Build history of the part. All positions in model axes, mm. A direction names the side the tool comes from. Give positions to 0.01 mm unless a question says otherwise; leave off trailing zeros. Loops run counter-clockwise (first coordinate to the right, second up) from the corner with the lowest first, then second, coordinate; pieces in that order, holes last. Notation, with made-up numbers: (40.5, 89.25) -> (46.5, 89.25) arc R30 cw to (46.5, 115.25) -> close; hole circle Ø7 at (39.5, -23). An arc over 180 degrees is marked (long way). Answer as a JSON object with one key per item and string values. Group by question number.
Q1. Band-saw the part on B-B, the plane z = 17. Count the separate pieces of the cut face and the enclosed holes in it, plus the area to 3 significant figures.
Q2. Two-plate mould, pull along X, no slides. Class faces 1 (the flat face through (112.867, -11, 13)), 2 (the flat face through (57.2, -26.2, 12.5)), 3 (the flat face through (127, -42, 25.4)), 4 (the cylindrical face through (-0.831, 67.892, 30.244)): pulls with the +X half, pulls with the -X half, needs draft (parallel to the pull), parting line crosses it, or undercut.
Q3. Wall check: probe 1 along Z at (x, y) = (220, -45.5); probe 2 along Y at (x, z) = (127.5, 11); probe 3 along Y at (x, z) = (140, 21). Give the ranges that are in metal, low to high. Write a range as from..to.
Q4. Drop flat-ended pins along their axis: pin 1 (20.5 mm diameter, centred on y = 0, z = 10.5, fed in from -X); pin 2 (8 mm diameter, centred on x = 116.5, z = 21, fed in from -Y); pin 3 (1.4 mm diameter, centred on y = -30.5, z = 15, fed in from +X); pin 4 (12 mm diameter, centred on x = 196, z = 32.5, fed in from -Y). Give the stop position or say it passes through.
Q5. Tool access for faces 5 (the flat face through (164, -42, 0)), 6 (the flat face through (230.488, -22, 13)), 7 (the flat face through (0, 0, 0)): list every direction of +Z, -Z, +X, -X, +Y, -Y with a clear straight run to the whole face (end or side of a thin tool).
Q6. Band-saw the part on C-C, the plane x = 234.5. Write the cut outline in (y, z), plus the area to 3 significant figures.
Q7. Band-saw the part on A-A, the plane x = 0. Write the cut outline in (y, z).
from build123d import *

# Parameters (mm, degrees)
F1_R     = 6.379673691
F3_W     = 4.8832285095
F3_H     = 45.7555688669
F3_H_2   = 32.2255445958
F4_DEPTH = 25.4
F6_DEPTH = 25.4


with BuildPart() as f2:
    # F2: sweep along a path in F0
    with BuildLine(Plane.YZ) as f2_path:
        Line((0, 0), (48.8668594837, 0))
        ThreePointArc((48.8668594837, 0), (57.8471156048, 3.7197438789), (61.5668594837, 12.7))
        Line((61.5668594837, 12.7), (61.5668594837, 47.304409945))
        ThreePointArc((61.5668594837, 47.304409945), (65.2866033626, 56.2846660661), (74.2668594837, 60.004409945))
        Line((74.2668594837, 60.004409945), (106.4591375947, 60.004409945))
    # F1 (on Front) → F2 (sweep)
    with BuildSketch(Plane.XZ):
        Circle(F1_R)
    sweep(path=f2_path.line)

    # F3 (on Top) → F4 (join)
    with BuildSketch(Plane.XY):
        Polygon((326.6327083111, 18.4751711786), (4.1886316997, 19.5212387724), (90.2807963532, -142.4016799862), align=None)
        Polygon((87.5756415589, -33.0956764519), (82.4007365874, -33.0956764519), (77.0470621713, -19.4245184088), (59.819333075, -19.4245184088), (54.5315210859, -33.0956764519), (49.4695231318, -33.0956764519), (66.4620292749, 10.0724399292), (70.6678156791, 10.0724399292), align=None, mode=Mode.SUBTRACT)
        with Locations((95.1921607853, -10.2178920185)):
            Rectangle(F3_W, F3_H, mode=Mode.SUBTRACT)
        with Locations((110.425199238, -10.2178920185)):
            Rectangle(F3_W, F3_H, mode=Mode.SUBTRACT)
        with Locations((125.6582376907, -16.982904154)):
            Rectangle(F3_W, F3_H_2, mode=Mode.SUBTRACT)
        with BuildLine():
            add(Edge.make_bspline(
                [(157.2204535583, -18.9822992567), (159.2339620381, -21.099305836), (159.2339620381, -24.3077469184)],
                knots=[0, 0, 0, 1, 1, 1], degree=2))
            add(Edge.make_bspline(
                [(159.2339620381, -24.3077469184), (159.2339620381, -28.8052097846), (155.8843871838, -31.2468240393)],
                knots=[0, 0, 0, 1, 1, 1], degree=2))
            add(Edge.make_bspline(
                [(155.8843871838, -31.2468240393), (152.5348123295, -33.6884382941), (146.4754690537, -33.6884382941)],
                knots=[0, 0, 0, 1, 1, 1], degree=2))
            add(Edge.make_bspline(
                [(146.4754690537, -33.6884382941), (140.067995807, -33.6884382941), (136.4831979994, -31.656111978)],
                knots=[0, 0, 0, 1, 1, 1], degree=2))
            Line((136.4831979994, -31.656111978), (136.4831979994, -27.1304223574))
            add(Edge.make_bspline(
                [(136.4831979994, -27.1304223574), (138.8072007776, -28.3065371237), (141.4652201494, -28.97927477)],
                knots=[0, 0, 0, 1, 1, 1], degree=2))
            add(Edge.make_bspline(
                [(141.4652201494, -28.97927477), (144.1232395211, -29.6520124163), (146.5977849894, -29.6520124163)],
                knots=[0, 0, 0, 1, 1, 1], degree=2))
            add(Edge.make_bspline(
                [(146.5977849894, -29.6520124163), (150.4178057502, -29.6520124163), (152.4736543616, -28.4335575184)],
                knots=[0, 0, 0, 1, 1, 1], degree=2))
            add(Edge.make_bspline(
                [(152.4736543616, -28.4335575184), (154.5295029731, -27.2151026206), (154.5295029731, -24.712330398)],
                knots=[0, 0, 0, 1, 1, 1], degree=2))
            add(Edge.make_bspline(
                [(154.5295029731, -24.712330398), (154.5295029731, -22.8305467719), (152.9017601366, -21.4944803975)],
                knots=[0, 0, 0, 1, 1, 1], degree=2))
            add(Edge.make_bspline(
                [(152.9017601366, -21.4944803975), (151.2740173, -20.158414023), (146.5319225624, -18.3330839057)],
                knots=[0, 0, 0, 1, 1, 1], degree=2))
            add(Edge.make_bspline(
                [(146.5319225624, -18.3330839057), (142.0344596962, -16.6582964786), (140.138562693, -15.4069103672)],
                knots=[0, 0, 0, 1, 1, 1], degree=2))
            add(Edge.make_bspline(
                [(140.138562693, -15.4069103672), (138.2426656898, -14.1555242559), (137.315887254, -12.570121551)],
                knots=[0, 0, 0, 1, 1, 1], degree=2))
            add(Edge.make_bspline(
                [(137.315887254, -12.570121551), (136.3891088181, -10.9847188461), (136.3891088181, -8.7830320036)],
                knots=[0, 0, 0, 1, 1, 1], degree=2))
            add(Edge.make_bspline(
                [(136.3891088181, -8.7830320036), (136.3891088181, -4.8406953071), (139.5975499005, -2.5590326605)],
                knots=[0, 0, 0, 1, 1, 1], degree=2))
            add(Edge.make_bspline(
                [(139.5975499005, -2.5590326605), (142.8059909829, -0.277370014), (148.3854794341, -0.277370014)],
                knots=[0, 0, 0, 1, 1, 1], degree=2))
            add(Edge.make_bspline(
                [(148.3854794341, -0.277370014), (153.5886111601, -0.277370014), (158.5659288509, -2.3943765933)],
                knots=[0, 0, 0, 1, 1, 1], degree=2))
            Line((158.5659288509, -2.3943765933), (156.8252789968, -6.3649400442))
            add(Edge.make_bspline(
                [(156.8252789968, -6.3649400442), (151.9796861598, -4.3702494006), (148.0373494633, -4.3702494006)],
                knots=[0, 0, 0, 1, 1, 1], degree=2))
            add(Edge.make_bspline(
                [(148.0373494633, -4.3702494006), (144.5654586732, -4.3702494006), (142.8012865238, -5.4569794446)],
                knots=[0, 0, 0, 1, 1, 1], degree=2))
            add(Edge.make_bspline(
                [(142.8012865238, -5.4569794446), (141.0371143744, -6.5437094886), (141.0371143744, -8.4537198691)],
                knots=[0, 0, 0, 1, 1, 1], degree=2))
            add(Edge.make_bspline(
                [(141.0371143744, -8.4537198691), (141.0371143744, -9.752150571), (141.7004431026, -10.6601111706)],
                knots=[0, 0, 0, 1, 1, 1], degree=2))
            add(Edge.make_bspline(
                [(141.7004431026, -10.6601111706), (142.3637718308, -11.5680717701), (143.8315630591, -12.3913521065)],
                knots=[0, 0, 0, 1, 1, 1], degree=2))
            add(Edge.make_bspline(
                [(143.8315630591, -12.3913521065), (145.2993542874, -13.2146324429), (149.4769139372, -14.7765128525)],
                knots=[0, 0, 0, 1, 1, 1], degree=2))
            add(Edge.make_bspline(
                [(149.4769139372, -14.7765128525), (155.2069450784, -16.8652926774), (157.2204535583, -18.9822992567)],
                knots=[0, 0, 0, 1, 1, 1], degree=2))
        make_face(mode=Mode.SUBTRACT)
        with BuildLine():
            add(Edge.make_bspline(
                [(123.6259113746, 5.4056165366), (122.8026310382, 6.2147834958), (122.8026310382, 7.8613441686)],
                knots=[0, 0, 0, 1, 1, 1], degree=2))
            add(Edge.make_bspline(
                [(122.8026310382, 7.8613441686), (122.8026310382, 9.5361315958), (123.6259113746, 10.3170718006)],
                knots=[0, 0, 0, 1, 1, 1], degree=2))
            add(Edge.make_bspline(
                [(123.6259113746, 10.3170718006), (124.449191711, 11.0980120054), (125.6911689042, 11.0980120054)],
                knots=[0, 0, 0, 1, 1, 1], degree=2))
            add(Edge.make_bspline(
                [(125.6911689042, 11.0980120054), (126.8672836704, 11.0980120054), (127.7187907612, 10.3029584234)],
                knots=[0, 0, 0, 1, 1, 1], degree=2))
            add(Edge.make_bspline(
                [(127.7187907612, 10.3029584234), (128.570297852, 9.5079048414), (128.570297852, 7.8613441686)],
                knots=[0, 0, 0, 1, 1, 1], degree=2))
            add(Edge.make_bspline(
                [(128.570297852, 7.8613441686), (128.570297852, 6.2147834958), (127.7187907612, 5.4056165366)],
                knots=[0, 0, 0, 1, 1, 1], degree=2))
            add(Edge.make_bspline(
                [(127.7187907612, 5.4056165366), (126.8672836704, 4.5964495774), (125.6911689042, 4.5964495774)],
                knots=[0, 0, 0, 1, 1, 1], degree=2))
            add(Edge.make_bspline(
                [(125.6911689042, 4.5964495774), (124.449191711, 4.5964495774), (123.6259113746, 5.4056165366)],
                knots=[0, 0, 0, 1, 1, 1], degree=2))
        make_face(mode=Mode.SUBTRACT)
        with BuildLine():
            add(Edge.make_bspline(
                [(191.0031741046, -4.7795373392), (194.9878509327, -9.2817046645), (194.9878509327, -16.9499729406)],
                knots=[0, 0, 0, 1, 1, 1], degree=2))
            add(Edge.make_bspline(
                [(194.9878509327, -16.9499729406), (194.9878509327, -24.8346463337), (191.0219919408, -29.2615423139)],
                knots=[0, 0, 0, 1, 1, 1], degree=2))
            add(Edge.make_bspline(
                [(191.0219919408, -29.2615423139), (187.056132949, -33.6884382941), (180.0558978602, -33.6884382941)],
                knots=[0, 0, 0, 1, 1, 1], degree=2))
            add(Edge.make_bspline(
                [(180.0558978602, -33.6884382941), (175.7277955203, -33.6884382941), (172.378220666, -31.656111978)],
                knots=[0, 0, 0, 1, 1, 1], degree=2))
            add(Edge.make_bspline(
                [(172.378220666, -31.656111978), (169.0286458116, -29.6237856619), (167.2033156944, -25.8319916554)],
                knots=[0, 0, 0, 1, 1, 1], degree=2))
            add(Edge.make_bspline(
                [(167.2033156944, -25.8319916554), (165.3779855771, -22.040197649), (165.3779855771, -16.9499729406)],
                knots=[0, 0, 0, 1, 1, 1], degree=2))
            add(Edge.make_bspline(
                [(165.3779855771, -16.9499729406), (165.3779855771, -9.0747084657), (169.3203222737, -4.6760392398)],
                knots=[0, 0, 0, 1, 1, 1], degree=2))
            add(Edge.make_bspline(
                [(169.3203222737, -4.6760392398), (173.2626589702, -0.277370014), (180.262894059, -0.277370014)],
                knots=[0, 0, 0, 1, 1, 1], degree=2))
            add(Edge.make_bspline(
                [(180.262894059, -0.277370014), (187.0184972765, -0.277370014), (191.0031741046, -4.7795373392)],
                knots=[0, 0, 0, 1, 1, 1], degree=2))
        make_face(mode=Mode.SUBTRACT)
        with BuildLine():
            Line((230.4876990377, -33.0956764519), (225.6044705282, -33.0956764519))
            Line((225.6044705282, -33.0956764519), (225.6044705282, -12.2455138755))
            add(Edge.make_bspline(
                [(225.6044705282, -12.2455138755), (225.6044705282, -8.3125860971), (223.8120716244, -6.3696445032)],
                knots=[0, 0, 0, 1, 1, 1], degree=2))
            add(Edge.make_bspline(
                [(223.8120716244, -6.3696445032), (222.0196727206, -4.4267029094), (218.1902430416, -4.4267029094)],
                knots=[0, 0, 0, 1, 1, 1], degree=2))
            add(Edge.make_bspline(
                [(218.1902430416, -4.4267029094), (213.1376540058, -4.4267029094), (210.7854244732, -7.1599936262)],
                knots=[0, 0, 0, 1, 1, 1], degree=2))
            add(Edge.make_bspline(
                [(210.7854244732, -7.1599936262), (208.4331949407, -9.893284343), (208.4331949407, -16.187850572)],
                knots=[0, 0, 0, 1, 1, 1], degree=2))
            Line((208.4331949407, -16.187850572), (208.4331949407, -33.0956764519))
            Line((208.4331949407, -33.0956764519), (203.5499664311, -33.0956764519))
            Line((203.5499664311, -33.0956764519), (203.5499664311, -0.8701318562))
            Line((203.5499664311, -0.8701318562), (207.5205298821, -0.8701318562))
            Line((207.5205298821, -0.8701318562), (208.310879005, -5.2829144592))
            Line((208.310879005, -5.2829144592), (208.5461019582, -5.2829144592))
            add(Edge.make_bspline(
                [(208.5461019582, -5.2829144592), (210.0515288591, -2.9024581723), (212.7565928215, -1.5899140931)],
                knots=[0, 0, 0, 1, 1, 1], degree=2))
            add(Edge.make_bspline(
                [(212.7565928215, -1.5899140931), (215.4616567839, -0.277370014), (218.7830048838, -0.277370014)],
                knots=[0, 0, 0, 1, 1, 1], degree=2))
            add(Edge.make_bspline(
                [(218.7830048838, -0.277370014), (224.6071252064, -0.277370014), (227.5474121221, -3.0859320758)],
                knots=[0, 0, 0, 1, 1, 1], degree=2))
            add(Edge.make_bspline(
                [(227.5474121221, -3.0859320758), (230.4876990377, -5.8944941377), (230.4876990377, -12.0761533492)],
                knots=[0, 0, 0, 1, 1, 1], degree=2))
            Line((230.4876990377, -12.0761533492), (230.4876990377, -33.0956764519))
        make_face(mode=Mode.SUBTRACT)
    extrude(amount=F4_DEPTH)

    # F5 (on face) → F6 (cut)
    with BuildSketch(Plane.XY.offset(25.4)):
        with BuildLine():
            add(Edge.make_bspline(
                [(97.6337750401, -70.9894448519), (101.7547711877, -65.7406254256), (109.5285345779, -55.8393591211), (123.9027278105, -73.6053108216), (107.611078169, -87.0535187852), (97.6337750401, -95.2894464135)],
                knots=[0, 0, 0, 0, 0.3042335189, 0.5738999278, 1, 1, 1, 1], degree=3))
            add(Edge.make_bspline(
                [(97.6337750401, -70.9894448519), (93.5127788924, -65.7406254256), (85.7390155022, -55.8393591211), (71.3648222696, -73.6053108216), (87.6564719111, -87.0535187852), (97.6337750401, -95.2894464135)],
                knots=[0, 0, 0, 0, 0.3042335189, 0.5738999278, 1, 1, 1, 1], degree=3))
        make_face()
    extrude(amount=-F6_DEPTH, mode=Mode.SUBTRACT)


solid = f2.part
Worked answers:
{
 "1": {"separate pieces": "2", "enclosed holes": "9", "area": "22,600 mm2"},
 "2": {"face 1": "undercut", "face 2": "undercut", "face 3": "needs draft", "face 4": "parting line crosses it"},
 "3": {"probe 1": "0..25.4", "probe 2": "-117.07..-33.1, -0.87..5.22, 10.49..19.12", "probe 3": "-108.56..-33.01, -28.56..-15.31, -2.29..19.08"},
 "4": {"pin 1": "x = -6.37", "pin 2": "y = -127.28", "pin 3": "x = 255.71", "pin 4": "through"},
 "5": {"face 5": "-Z, +X, +Y, -Y", "face 6": "+Z, -Z", "face 7": "+Z, -Z, -X, -Y"},
 "6": {"outline": "(-44.24, 0) -> (18.77, 0) -> (18.77, 25.4) -> (-44.24, 25.4) -> close", "area": "1,600 mm2"},
 "7": {"outline": "(0, -6.38) -> (48.87, -6.38) arc R19.08 ccw to (67.95, 12.7) -> (67.95, 47.3) arc R6.32 cw to (74.27, 53.62) -> (106.46, 53.62) -> (106.46, 66.38) -> (74.27, 66.38) arc R19.08 ccw to (55.19, 47.3) -> (55.19, 12.7) arc R6.32 cw to (48.87, 6.38) -> (0, 6.38) -> close"}
}
